CAD build for the part. Positions are in the model's coordinates, mm. Give positions to 0.01 mm unless a question says otherwise; leave off trailing zeros. Order: outer loops, then holes, each group sorted by start corner. A loop starts at its lowest first (then second) coordinate and runs counter-clockwise, first axis right, second up.
Item 1: Band-saw the part on D-D on z = 3.5. Give the cut face in (x, y).
Item 2: Band-saw the part on B-B on y = 0.35. Give the cut face in (x, z), plus the area to 3 significant figures.
Item 3: Flat gauge pins, fed straight in: P1, Ø0.5, axis at x = 3, y = 0.5, coming from the -Z side; P2, Ø2, axis at x = 0, z = 5.5, coming from the +Y side. Where does each tip first touch, or does it go through?
Item 4: Wall check: L1, parallel to X at y = 0.7, z = -1; L2, parallel to Z at x = -5.5, y = 0.5; L3, parallel to Z at x = -4, y = 0.7. Give the ranges that are in metal, low to high.
Item 5: Band-saw the part on C-C on x = 0. Give the cut face in (y, z).
Item 6: Band-saw the part on A-A on z = 0. Give the cut face in (x, y).
```python
from build123d import *

# Parameters (mm, degrees)
SKETCH1_R           = 7.26
BOSS_EXTRUDE1_DEPTH = 1
CUT_EXTRUDE1_DEPTH  = 2
CUT_EXTRUDE2_DEPTH  = 2
CUT_EXTRUDE3_DEPTH  = 2
FILLET1_R           = 0.3


with BuildPart() as part:
    # Sketch1 → Boss-Extrude1 (new body)
    with BuildSketch(Plane(origin=(0, 0, 0), x_dir=(1, 0, 0), z_dir=(0, 1, 0))):
        Circle(SKETCH1_R)
    extrude(amount=BOSS_EXTRUDE1_DEPTH)

    # Sketch2 → Cut-Extrude1 (cut, through all)
    with BuildSketch(Plane(origin=(0, 1, 0), x_dir=(1, 0, 0), z_dir=(0, 1, 0))):
        with BuildLine():
            Line((-1.5, 7.103351322), (-1.5, 6))
            Line((-1.5, 6), (1.5, 6))
            Line((1.5, 6), (1.5, 7.103351322))
            ThreePointArc((1.5, 7.103351322), (0, 7.26), (-1.5, 7.103351322))
        make_face()
    extrude(amount=-CUT_EXTRUDE1_DEPTH, mode=Mode.SUBTRACT)

    # Sketch3 → Cut-Extrude2 (cut, through all)
    with BuildSketch(Plane(origin=(0, 1, 0), x_dir=(1, 0, 0), z_dir=(0, 1, 0))):
        with BuildLine():
            Line((2, 1.5), (6, 1.5))
            Line((6, 1.5), (6, -1.5))
            Line((6, -1.5), (2, -1.5))
            ThreePointArc((2, -1.5), (0, -2.5), (-2, -1.5))
            Line((-2, -1.5), (-6, -1.5))
            Line((-6, -1.5), (-6, 1.5))
            Line((-6, 1.5), (-2, 1.5))
            ThreePointArc((-2, 1.5), (0, 2.5), (2, 1.5))
        make_face()
    extrude(amount=-CUT_EXTRUDE2_DEPTH, mode=Mode.SUBTRACT)

    # Sketch4 → Cut-Extrude3 (cut, through all)
    with BuildSketch(Plane(origin=(0, 1, 0), x_dir=(1, 0, 0), z_dir=(0, 1, 0))):
        with BuildLine():
            Line((-1.8, -6.4), (-1.8, -7.033320695))
            ThreePointArc((-1.8, -7.033320695), (0, -7.26), (1.8, -7.033320695))
            Line((1.8, -7.033320695), (1.8, -6.4))
            ThreePointArc((1.8, -6.4), (0, -4.6), (-1.8, -6.4))
        make_face()
    extrude(amount=-CUT_EXTRUDE3_DEPTH, mode=Mode.SUBTRACT)

    # Fillet1
    fillet1_edges = [part.edges().sort_by_distance(p)[0] for p in [
        (1.5, 0.5, -6),
        (-1.5, 0.5, -6),
    ]]
    fillet(fillet1_edges, radius=FILLET1_R)


solid = part.part
```
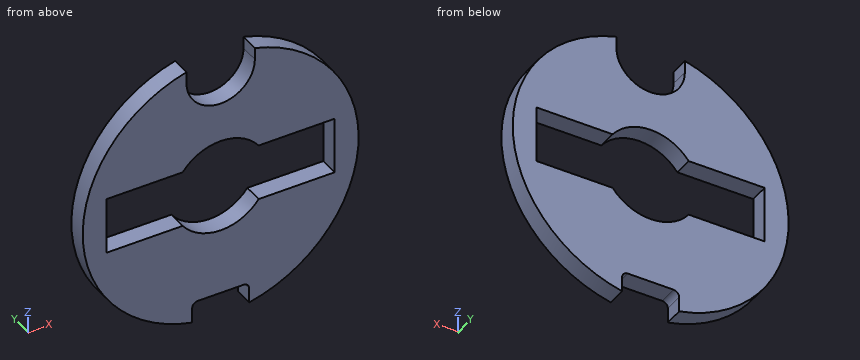
The answers:
1. outline: (-6.36, 0) - (6.36, 0) - (6.36, 1) - (-6.36, 1) - close
2. outline: (-1.8, 6.4) - (-1.8, 7.03) arc R7.26 ccw to (-1.5, -7.1) - (-1.5, -6.3) arc R0.3 cw to (-1.2, -6) - (1.2, -6) arc R0.3 cw to (1.5, -6.3) - (1.5, -7.1) arc R7.26 ccw to (1.8, 7.03) - (1.8, 6.4) arc R1.8 cw to start; hole (-6, -1.5) - (-2, -1.5) arc R2.5 ccw to (2, -1.5) - (6, -1.5) - (6, 1.5) - (2, 1.5) arc R2.5 ccw to (-2, 1.5) - (-6, 1.5) - close
2. area: 112 mm2
3. P1: stops at z = -6.72
3. P2: stops at y = 1
4. L1: x = -7.19 to -6, 6 to 7.19
4. L2: z = -4.74 to -1.5, 1.5 to 4.74
4. L3: z = -6.06 to -1.5, 1.5 to 6.06
5. outline: (0, -6) - (1, -6) - (1, -2.5) - (0, -2.5) - close; (0, 2.5) - (1, 2.5) - (1, 4.6) - (0, 4.6) - close
6. outline: (-7.26, 0) - (-6, 0) - (-6, 1) - (-7.26, 1) - close; (6, 0) - (7.26, 0) - (7.26, 1) - (6, 1) - close
